Build history of the part. All positions in model axes, mm. Face numbers are marked on the shaded views. A direction names the side the tool comes from. Give positions to 0.01 mm unless a question says otherwise; leave off trailing zeros. Loops run counter-clockwise (first coordinate to the right, second up) from the corner with the lowest first, then second, coordinate; pieces in that order, holes last. Notation, with made-up numbers: (58.5, 25) -> (94.5, 25) arc R24 ccw to (94.5, 35) -> close; hole circle Ø10 at (26.5, -21.75). An arc over 180 degrees is marked (long way). Answer in a Markdown table with one row per item. Add a question column.
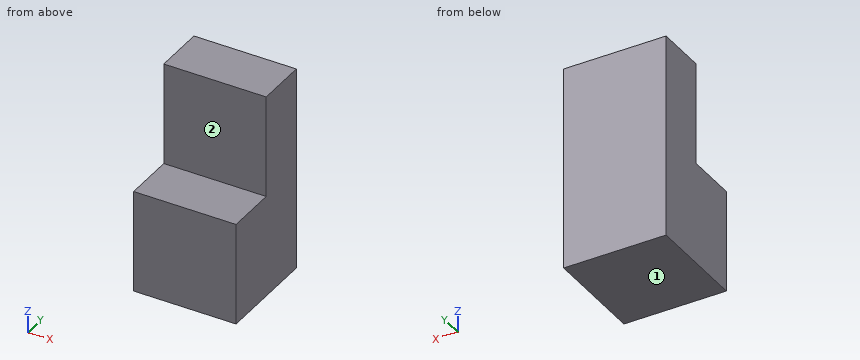
from build123d import *

# Parameters (mm, degrees)
F0_W     = 15.6972
F0_H     = 15.6972
F1_DEPTH = 7.8486
F2_DEPTH = 7.8486


with BuildPart() as f1:
    # F0 (on Front) → F1 (new body)
    with BuildSketch(Plane.XZ):
        with Locations((0.617838, -29.792661)):
            Rectangle(F0_W, F0_H)
    extrude(amount=F1_DEPTH)

    # F0 (on Front) → F2 (join)
    with BuildSketch(Plane.XZ):
        with Locations((0.617838, -14.095461)):
            Rectangle(F0_W, F0_H)
        with Locations((0.617838, -29.792661)):
            Rectangle(F0_W, F0_H)
    extrude(amount=-F2_DEPTH)


solid = f1.part
(1) 3-axis set-ups, long thin cutter, end or side, ignore diameter. For the marked faces 1 and 2: which of +Z, -Z, +X, -X, +Y, -Y reach the whole face in a straight line?
(2) Saw through at B-B, the plane y = -3.75. List the corners of the cut face in (x, z).
(3) Saw through at C-C, the plane z = -19. List the corners of the cut face in (x, y), then the cut area to 3 significant figures.
(4) Wall check: line 1 along Y through (x, z) = (1.5, -16); line 2 along Z through (x, y) = (2, -5.75). Give the ranges that are in metal, low to high. Write a range as from..to.
(5) Saw through at A-A, the plane x = 1.5. List the corners of the cut face in (y, z).
(6) Flat gauge pins, fed straight in: pin 1 Ø5 at (x, z) = (3, -16.5) entering from -Y; pin 2 Ø1 at (y, z) = (-5, -20.5) entering from -X; pin 3 Ø6.5 at (x, y) = (4, -6) entering from +Z. Where does each tip first touch, or does it go through?
Worked answers:
| question | item | result |
|---|---|---|
| 1 | face 1 | -Z, +X, -X, +Y, -Y |
| 1 | face 2 | +Z, +X, -X, -Y |
| 2 | outline | (-7.23, -37.64) -> (8.47, -37.64) -> (8.47, -21.94) -> (-7.23, -21.94) -> close |
| 3 | outline | (-7.23, 0) -> (8.47, 0) -> (8.47, 7.85) -> (-7.23, 7.85) -> close |
| 3 | area | 123 mm^2 |
| 4 | line 1 | 0..7.85 |
| 4 | line 2 | -37.64..-21.94 |
| 5 | outline | (-7.85, -37.64) -> (7.85, -37.64) -> (7.85, -6.25) -> (0, -6.25) -> (0, -21.94) -> (-7.85, -21.94) -> close |
| 6 | pin 1 | y = 0 |
| 6 | pin 2 | through |
| 6 | pin 3 | z = -21.94 |
